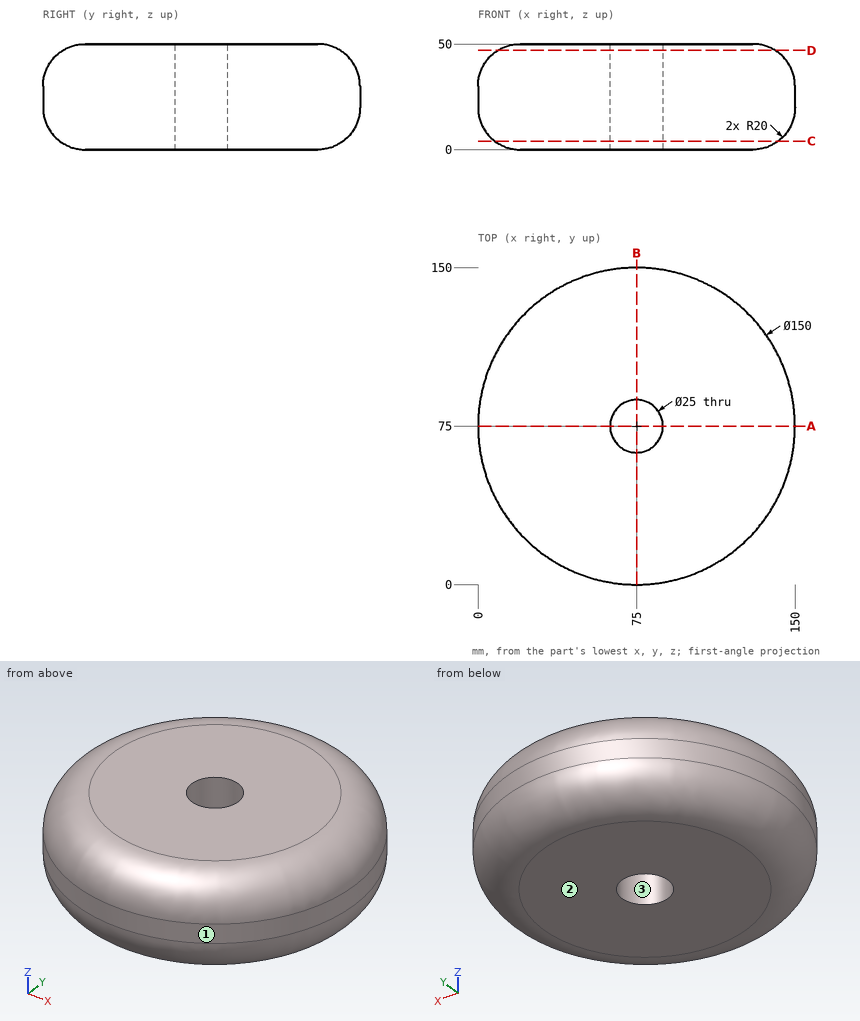
Drawing for the job (mm, zero at the part's lowest x, y, z). Round coordinates to 2 decimals unless told otherwise and drop trailing zeros. Loops run counter-clockwise (first coordinate to the right, second up) from the corner with the lowest first, then second, coordinate; pieces in that order, holes last. Notation, with made-up numbers: (88.25, 68.25) -> (117.25, 68.25) arc R24 cw to (117.25, 95.25) -> close; hole circle Ø5 at (-18, -6.75). An arc over 180 degrees is marked (long way). Use one line per item in the form item = value. Start each with the question number.
Item 1: Drill centre lines: line 1 along Y through (x, z) = (75, 23.5); line 2 along Y through (x, z) = (69.5, 43.5); line 3 along X through (y, z) = (70, 7.5). Where is each one in solid material? Low to high.
Item 2: Band-saw the part on D-D (z = 47). List the corners of the cut face in (x, y), plus the area to 3 significant figures.
Item 3: Band-saw the part on C-C (z = 4). List the corners of the cut face in (x, y).
Item 4: Two-plate mould, pull along X, no slides. Class the marked faces 1, 2 and 3: released by +X, released by -X, zero draft, split by the parting line, or undercut.
Item 5: Band-saw the part on A-A (y = 75). List the corners of the cut face in (x, z).
Item 6: Drop flat-ended pins along their axis: pin 1 Ø8 at (x, z) = (46.5, 12.5) entering from -Y; pin 2 Ø12 at (y, z) = (57, 18) entering from -X; pin 3 Ø6 at (y, z) = (56.5, 36) entering from -X; pin 4 Ø15 at (x, y) = (75, 75) entering from +Z. Give the stop position or say it passes through.
Data:
q1.line_1 = 0 to 62.5, 87.5 to 150
q1.line_2 = 5.46 to 63.78, 86.22 to 144.54
q1.line_3 = 4.56 to 63.54, 86.46 to 145.44
q2.outline = circle Ø131.07 at (75, 75); hole circle Ø25 at (75, 75)
q2.area = 13,000 mm^2
q3.outline = circle Ø134 at (75, 75); hole circle Ø25 at (75, 75)
q4.face_1 = split by the parting line
q4.face_2 = zero draft
q4.face_3 = undercut
q5.outline = (0, 20) arc R20 ccw to (20, 0) -> (62.5, 0) -> (62.5, 50) -> (20, 50) arc R20 ccw to (0, 30) -> close; (87.5, 0) -> (130, 0) arc R20 ccw to (150, 20) -> (150, 30) arc R20 ccw to (130, 50) -> (87.5, 50) -> close
q6.pin_1 = 5.1
q6.pin_2 = 1
q6.pin_3 = 2.2
q6.pin_4 = through
